Can you work these out from the model? Positions are in its coordinate system, mm. A direction names the side the tool comes from. Give positions to 0.01 mm unless a question says otherwise; leave off trailing zeros. Loops run counter-clockwise (first coordinate to the right, second up) from the corner with the lowest first, then second, coordinate; pieces in that order, holes last. Notation, with made-up numbers: M 29,74 L 67,74 A24 ccw 67,108 Z; hole C 38.25,64.5 d2. An arc over 180 degrees is marked long. Answer as a JSON object with one key per item and string values.
```python
from build123d import *

# Parameters (mm, degrees)
SKETCH1_R           = 14
BOSS_EXTRUDE1_DEPTH = 19
BOSS_EXTRUDE2_START = -2
SKETCH4_R           = 2
BOSS_EXTRUDE2_DEPTH = 2
SKETCH5_R           = 4.5
BOSS_EXTRUDE3_DEPTH = 1.5
SKETCH6_R           = 2.5
BOSS_EXTRUDE4_DEPTH = 2.5
SKETCH7_R           = 1.5
BOSS_EXTRUDE5_DEPTH = 6
SKETCH8_W           = 12
SKETCH8_H           = 2
CUT_EXTRUDE1_DEPTH  = 4


with BuildPart() as part:
    # Sketch1 → Boss-Extrude1 (new body)
    with BuildSketch(Plane(origin=(0, 0, 0), x_dir=(1, 0, 0), z_dir=(0, 1, 0))):
        Circle(SKETCH1_R)
        with BuildLine():
            Line((-7.3, -11.94612908), (-7.3, -17))
            Line((-7.3, -17), (0, -17))
            Line((0, -17), (7.3, -17))
            Line((7.3, -17), (7.3, -11.94612908))
            ThreePointArc((7.3, -11.94612908), (0, -14), (-7.3, -11.94612908))
        make_face()
    extrude(amount=BOSS_EXTRUDE1_DEPTH)

    # Sketch4 → Boss-Extrude2 (add)
    # profile 1 of 2: a face of its own
    with BuildSketch(Plane(origin=(0, 19, 0), x_dir=(1, 0, 0), z_dir=(0, 1, 0)).offset(BOSS_EXTRUDE2_START)):
        with BuildLine():
            ThreePointArc((-17.5, 3.5), (-21, 0), (-17.5, -3.5))
            Line((-17.5, -3.5), (-13.555441712, -3.5))
            ThreePointArc((-13.555441712, -3.5), (-14, 0), (-13.555441712, 3.5))
            Line((-13.555441712, 3.5), (-17.5, 3.5))
        make_face()
        with Locations(Location((-17.5, 0, 0), (0, 0, 270))):
            Circle(SKETCH4_R, mode=Mode.SUBTRACT)
    # profile 2 of 2: a face of its own
    with BuildSketch(Plane(origin=(0, 19, 0), x_dir=(1, 0, 0), z_dir=(0, 1, 0)).offset(BOSS_EXTRUDE2_START)):
        with BuildLine():
            Line((17.5, 3.5), (13.555441712, 3.5))
            ThreePointArc((13.555441712, 3.5), (14, 0), (13.555441712, -3.5))
            Line((13.555441712, -3.5), (17.5, -3.5))
            ThreePointArc((17.5, -3.5), (21, 0), (17.5, 3.5))
        make_face()
        with Locations(Location((17.5, 0, 0), (0, 0, 270))):
            Circle(SKETCH4_R, mode=Mode.SUBTRACT)
    extrude(amount=BOSS_EXTRUDE2_DEPTH)

    # Sketch5 → Boss-Extrude3 (add)
    with BuildSketch(Plane(origin=(0, 19, 0), x_dir=(1, 0, 0), z_dir=(0, 1, 0))):
        with Locations(Location((0, 8, 0), (0, 0, 270))):
            Circle(SKETCH5_R)
    extrude(amount=BOSS_EXTRUDE3_DEPTH)

    # Sketch6 → Boss-Extrude4 (add)
    with BuildSketch(Plane(origin=(0, 20.5, 0), x_dir=(1, 0, 0), z_dir=(0, 1, 0))):
        with Locations(Location((0, 8, 0), (0, 0, 270))):
            Circle(SKETCH6_R)
    extrude(amount=BOSS_EXTRUDE4_DEPTH)

    # Sketch7 → Boss-Extrude5 (add)
    with BuildSketch(Plane(origin=(0, 23, 0), x_dir=(1, 0, 0), z_dir=(0, 1, 0))):
        with Locations(Location((0, 8, 0), (0, 0, 270))):
            Circle(SKETCH7_R)
    extrude(amount=BOSS_EXTRUDE5_DEPTH)

    # Sketch8 → Cut-Extrude1 (cut)
    with BuildSketch(Plane.XY.offset(17)):
        with Locations((0, 15.332469826)):
            Rectangle(SKETCH8_W, SKETCH8_H)
    extrude(amount=-CUT_EXTRUDE1_DEPTH, mode=Mode.SUBTRACT)


solid = part.part
```
1) Suppose I cut it at A-A, the plane z = 0. Write out the boundary of the cut face in (x, y), and give its area (3 significant figures).
Answer list:
{"outline": "M -21,17 L -19.5,17 L -19.5,19 L -21,19 Z; M -15.5,17 L -14,17 L -14,0 L 14,0 L 14,17 L 15.5,17 L 15.5,19 L -15.5,19 Z; M 19.5,17 L 21,17 L 21,19 L 19.5,19 Z", "area": "544 mm^2"}
2) Suppose I cut it at C-C, the plane x = -16. Write out the boundary of the cut face in (y, z), and give its area (3 significant figures).
Answer list:
{"outline": "M 17,-3.5 L 19,-3.5 L 19,-1.32 L 17,-1.32 Z; M 17,1.32 L 19,1.32 L 19,3.5 L 17,3.5 Z", "area": "8.71 mm^2"}
3) Suppose I cut it at B-B, the plane x = 0. Write out the boundary of the cut face in (y, z).
Answer list:
{"outline": "M 0,-14 L 19,-14 L 19,-12.5 L 20.5,-12.5 L 20.5,-10.5 L 23,-10.5 L 23,-9.5 L 29,-9.5 L 29,-6.5 L 23,-6.5 L 23,-5.5 L 20.5,-5.5 L 20.5,-3.5 L 19,-3.5 L 19,17 L 16.33,17 L 16.33,13 L 14.33,13 L 14.33,17 L 0,17 Z"}
4) For faces 4 (the flat face through (-16, 18, 3.5)), 5 (the flat face through (0, 14.332, 15)), 6 (the cylindrical face through (0.1, 21.7, -10.5)), 7 (the cylindrical face through (0.51, 9.37, -13.99)), which set-ups out of +Z, -Z, +X, -X, +Y, -Y let a thin tool reach every point of the face, with its end or its side?
Answer list:
{"face 4": "+Z, -X, +Y, -Y", "face 5": "+Z", "face 6": "+Y", "face 7": "-Y"}
5) Suppose I cut it at D-D, the plane z = -5. Write out the boundary of the cut face in (x, y).
Answer list:
{"outline": "M -13.08,0 L 13.08,0 L 13.08,19 L 3.35,19 L 3.35,20.5 L -3.35,20.5 L -3.35,19 L -13.08,19 Z"}
6) Please list where these lines run through material, in increasing order: line 1 along X through (y, z) = (18.15, 0); line 2 along Y through (x, z) = (10.5, 4); line 3 along Y through (x, z) = (5, 14.5). Write a range as from..to.
Answer list:
{"line 1": "-21..-19.5, -15.5..15.5, 19.5..21", "line 2": "0..19", "line 3": "0..14.33, 16.33..19"}
7) If we mould it in two halves opening along X, with no side actions, what happens to faces 1 (the flat face through (7.3, 9, 15)), 2 (the cylindrical face through (19.483, 17.986, -0.26)), 3 (the flat face through (16, 17, -2))? For each: +X half, -X half, draft (parallel to the pull), parting line (faces both ways), or undercut.
Answer list:
{"face 1": "+X half", "face 2": "undercut", "face 3": "draft"}
8) Will these pins go through, and if not, where does the flat tip stop? pin 1 Ø2 at (x, z) = (-2, 14.5) entering from +Y; pin 2 Ø6 at (y, z) = (7, -4) entering from +X; pin 3 Ø2 at (y, z) = (11, 7.5) entering from -X.
Answer list:
{"pin 1": "y = 19", "pin 2": "x = 13.96", "pin 3": "x = -12.4"}
